from build123d import *

# Parameters (mm, degrees)
BOSS_EXTRUDE2_DEPTH = 213
SKETCH2_W           = 57.4
SKETCH2_H           = 19.4
BOSS_EXTRUDE3_DEPTH = 2
FILLET2_R           = 4
SKETCH3_R           = 11.35
CUT_EXTRUDE1_DEPTH  = 59


with BuildPart() as part:
    # Sketch1 → Boss-Extrude2 (new body)
    with BuildSketch(Plane.XY):
        Polygon((-24.7, 0.2), (0, 0.2), (0, 5.2), (-28.7, 5.2), (-28.7, -14.2), (-16.7, -14.2), (-16.7, -10), (-16.7, -5.2), (-20.3, -5.2), (-20.3, -10.2), (-24.7, -10.2), align=None)
        Polygon((0, 5.2), (0, 0.2), (24.7, 0.2), (24.7, -10.2), (20.3, -10.2), (20.3, -5.2), (16.7, -5.2), (16.7, -10), (16.7, -14.2), (28.7, -14.2), (28.7, 5.2), align=None)
    extrude(amount=BOSS_EXTRUDE2_DEPTH)

    # Sketch2 → Boss-Extrude3 (add)
    with BuildSketch(Plane(origin=(0, 0, 0), x_dir=(-1, 0, 0), z_dir=(0, 0, -1))):
        with Locations((0, -4.5)):
            Rectangle(SKETCH2_W, SKETCH2_H)
    extrude(amount=BOSS_EXTRUDE3_DEPTH)

    # Fillet2
    fillet2_edges = [part.edges().sort_by_distance(p)[0] for p in [
        (-28.7, -14.2, 105.5),
        (-28.7, 5.2, 105.5),
        (28.7, 5.2, 105.5),
        (28.7, -14.2, 105.5),
    ]]
    fillet(fillet2_edges, radius=FILLET2_R)

    # Sketch3 → Cut-Extrude1 (cut)
    with BuildSketch(Plane(origin=(0, 5.2, 0), x_dir=(1, 0, 0), z_dir=(0, 1, 0))):
        with Locations(Location((0, -31.5, 0), (0, 0, 180))):
            Circle(SKETCH3_R)
        with Locations(Location((0, -106.5, 0), (0, 0, 180))):
            Circle(SKETCH3_R)
        with Locations(Location((0, -181.5, 0), (0, 0, 180))):
            Circle(SKETCH3_R)
    extrude(amount=-CUT_EXTRUDE1_DEPTH, mode=Mode.SUBTRACT)


solid = part.part
Work out the finished part from the listing and answer in its coordinate system (mm). A direction names the side the tool comes from. Give positions to 0.01 mm unless a question says otherwise; leave off trailing zeros. Loops run counter-clockwise (first coordinate to the right, second up) from the corner with the lowest first, then second, coordinate; pieces in that order, holes last. Notation, with made-up numbers: M -17,73.25 L -4,73.25 A17 cw -4,103.25 Z; hole C 74.25,-15 d3. An arc over 180 degrees is marked long. Use CSV: the item, a comma, the result in double quotes.
1) Consider L1, parallel to Z at x = 0, y = 2.25; L2, parallel to X at y = -7, z = 134; L3, parallel to Y at x = 20, z = 179. Determine where each line is inside the solid, lowest interval first.
Answer:
L1,"-2 to 20.15, 42.85 to 95.15, 117.85 to 170.15, 192.85 to 213"
L2,"-28.7 to -24.7, -20.3 to -16.7, 16.7 to 20.3, 24.7 to 28.7"
L3,"-14.2 to -5.2, 0.2 to 5.2"
2) Find section B-B on z = 31.5. Write down the section's boundary in (x, y).
Answer:
outline,"M -28.7,-10.2 A4 ccw -24.7,-14.2 L -16.7,-14.2 L -16.7,-5.2 L -20.3,-5.2 L -20.3,-10.2 L -24.7,-10.2 L -24.7,0.2 L -11.35,0.2 L -11.35,5.2 L -24.7,5.2 A4 ccw -28.7,1.2 Z; M 11.35,0.2 L 24.7,0.2 L 24.7,-10.2 L 20.3,-10.2 L 20.3,-5.2 L 16.7,-5.2 L 16.7,-14.2 L 24.7,-14.2 A4 ccw 28.7,-10.2 L 28.7,1.2 A4 ccw 24.7,5.2 L 11.35,5.2 Z"
3) Find section A-A on x = 0. Write down the section's boundary in (y, z), plus the area to 3 significant figures.
Answer:
outline,"M -14.2,-2 L 5.2,-2 L 5.2,20.15 L 0.2,20.15 L 0.2,0 L -14.2,0 Z; M 0.2,42.85 L 5.2,42.85 L 5.2,95.15 L 0.2,95.15 Z; M 0.2,117.85 L 5.2,117.85 L 5.2,170.15 L 0.2,170.15 Z; M 0.2,192.85 L 5.2,192.85 L 5.2,213 L 0.2,213 Z"
area,"763 mm^2"
4) Given P1, Ø5, axis at x = -12, z = 69, coming from the -Y side; P2, Ø4.5, axis at x = 5.5, y = -7.5, coming from the +Z side, each flat-ended and moving along its own axis, determine where each tip first touches the part or whether it passes through.
Answer:
P1,"y = 0.2"
P2,"z = 0"
5) Find section C-C on y = -7.5. Write down the section's boundary in (x, z).
Answer:
outline,"M -28.7,-2 L 28.7,-2 L 28.7,213 L 24.7,213 L 24.7,0 L 20.3,0 L 20.3,213 L 16.7,213 L 16.7,0 L -16.7,0 L -16.7,213 L -20.3,213 L -20.3,0 L -24.7,0 L -24.7,213 L -28.7,213 Z"
6) Find section D-D on z = 79.5. Write down the section's boundary in (x, y), plus the area to 3 significant figures.
Answer:
outline,"M -28.7,-10.2 A4 ccw -24.7,-14.2 L -16.7,-14.2 L -16.7,-5.2 L -20.3,-5.2 L -20.3,-10.2 L -24.7,-10.2 L -24.7,0.2 L 24.7,0.2 L 24.7,-10.2 L 20.3,-10.2 L 20.3,-5.2 L 16.7,-5.2 L 16.7,-14.2 L 24.7,-14.2 A4 ccw 28.7,-10.2 L 28.7,1.2 A4 ccw 24.7,5.2 L -24.7,5.2 A4 ccw -28.7,1.2 Z"
area,"488 mm^2"
7) Determine the mould class of faces 1 (the flat face through (0, 2, 213)), 2 (the cylindrical face through (27.559, 3.997, 107.005)), 3 (the flat face through (23, -10.2, 105)) for opening direction Y: released by +Y, released by -Y, zero draft, split by the parting line, or undercut.
Answer:
face 1,"zero draft"
face 2,"released by +Y"
face 3,"undercut"
8) Which of the six approach directions +Z, -Z, +X, -X, +Y, -Y give full straight-line access (tool end or side, diameter ignored) to faces 4 (the cylindrical face through (-27.497, -13.059, 103.995)), 5 (the flat face through (16.7, -10, 105)), 6 (the flat face through (-22, -10.2, 105))?
Answer:
face 4,"+Z, -Z, -X, -Y"
face 5,"+Z, -Y"
face 6,"+Z"
